```python
from build123d import *

# Parameters (mm, degrees)
SKETCH_1_W          = 15
SKETCH_1_H          = 15
EXTRUDE_1_DEPTH     = 253
SKETCH_2_W          = 11
SKETCH_2_H          = 11
CUT_EXTRUDE_1_DEPTH = 253
SKETCH_3_R          = 1.5
CUT_EXTRUDE_2_DEPTH = 15
SKETCH_4_R          = 1.5
CUT_EXTRUDE_3_DEPTH = 15
SKETCH_5_R          = 2.5
CUT_EXTRUDE_4_DEPTH = 15


with BuildPart() as part:
    # 草图1 → 凸台-拉伸1 (new body)
    with BuildSketch(Plane(origin=(0, 0, 0), x_dir=(1, 0, 0), z_dir=(0, 1, 0))):
        Rectangle(SKETCH_1_W, SKETCH_1_H)
    extrude(amount=EXTRUDE_1_DEPTH)

    # 草图2 → 切除-拉伸1 (cut)
    with BuildSketch(Plane(origin=(0, 253, 0), x_dir=(1, 0, 0), z_dir=(0, 1, 0))):
        Rectangle(SKETCH_2_W, SKETCH_2_H)
    extrude(amount=-CUT_EXTRUDE_1_DEPTH, mode=Mode.SUBTRACT)

    # 草图3 → 切除-拉伸2 (cut)
    with BuildSketch(Plane(origin=(7.5, 0, 0), x_dir=(0, 0, -1), z_dir=(1, 0, 0))):
        with Locations((0, 17.5)):
            Circle(SKETCH_3_R)
        with Locations((0, 37.5)):
            Circle(SKETCH_3_R)
        with Locations((0, 57.5)):
            Circle(SKETCH_3_R)
    extrude(amount=-CUT_EXTRUDE_2_DEPTH, mode=Mode.SUBTRACT)

    # 草图4 → 切除-拉伸3 (cut)
    with BuildSketch(Plane(origin=(0, 0, -7.5), x_dir=(-1, 0, 0), z_dir=(0, 0, -1))):
        with Locations((0, 25.5)):
            Circle(SKETCH_4_R)
    extrude(amount=-CUT_EXTRUDE_3_DEPTH, mode=Mode.SUBTRACT)

    # 草图5 → 切除-拉伸4 (cut)
    with BuildSketch(Plane(origin=(0, 0, -7.5), x_dir=(-1, 0, 0), z_dir=(0, 0, -1))):
        with Locations((0, 213)):
            Circle(SKETCH_5_R)
        with Locations((0, 183)):
            Circle(SKETCH_5_R)
    extrude(amount=-CUT_EXTRUDE_4_DEPTH, mode=Mode.SUBTRACT)


solid = part.part
```
Work out the finished part from the listing and answer in its coordinate system (mm). A direction names the side the tool comes from. Coordinates: 2 decimals unless noted, no trailing zeros. Loops run counter-clockwise (first coordinate to the right, second up) from the corner with the lowest first, then second, coordinate; pieces in that order, holes last. Notation, with made-up numbers: (-5.75, 63.25) -> (47.25, 63.25) arc R22 cw to (47.25, 97.25) -> close; hole circle Ø11 at (66, 56). An arc over 180 degrees is marked (long way). Answer as CSV lines item,"result".
Q1. A tool of negligible diameter and unlimited length cuts with its end or side. For faces 5 (the face through (0, 128, -5.5)), 6 (the face through (-7.5, 125, 0)), from which of +Z, -Z, +X, -X, +Y, -Y can it reach the whole face along a straight path? Write none if from no direction.
Findings:
face 5,"+Y, -Y"
face 6,"+Z, -Z, -X, +Y, -Y"
Q2. For a pull along Z with two mould halves and no side action, classify faces 1 (the face through (0.33, 215.48, -6.51)), 2 (the face through (0, 125, -7.5)), 3 (the face through (0, 125, 7.5)), 4 (the face through (-5.5, 128, 0)) as +Z half, -Z half, draft (parallel to the pull), parting line (faces both ways), or undercut.
Findings:
face 1,"draft"
face 2,"-Z half"
face 3,"+Z half"
face 4,"undercut"
Q3. Find the intervals of material crossed by probe 1 along Y at (x, z) = (0, -6.45); probe 2 along Y at (x, z) = (6, 0); probe 3 along Z at (x, y) = (0.5, 84), in increasing order.
Findings:
probe 1,"y = 0 to 24, 27 to 180.5, 185.5 to 210.5, 215.5 to 253"
probe 2,"y = 0 to 16, 19 to 36, 39 to 56, 59 to 253"
probe 3,"z = -7.5 to -5.5, 5.5 to 7.5"
Q4. The part is cut by section A-A on y = 183. Write down the section's boundary in (x, z), and give its area (3 significant figures).
Findings:
outline,"(-7.5, -7.5) -> (-2.5, -7.5) -> (-2.5, -5.5) -> (-5.5, -5.5) -> (-5.5, 5.5) -> (-2.5, 5.5) -> (-2.5, 7.5) -> (-7.5, 7.5) -> close; (2.5, -7.5) -> (7.5, -7.5) -> (7.5, 7.5) -> (2.5, 7.5) -> (2.5, 5.5) -> (5.5, 5.5) -> (5.5, -5.5) -> (2.5, -5.5) -> close"
area,"84.0 mm²"
